```python
from build123d import *


with BuildPart() as part:
    # Esquisse1 → Révolution1 (revolve)
    with BuildSketch(Plane.XY):
        with BuildLine():
            Line((143.396454905, 12.7), (142.494, 12.7))
            Line((142.494, 12.7), (142.494, 0))
            Line((142.494, 0), (130.048, 0))
            Line((130.048, 0), (130.048, 38.1))
            Line((130.048, 38.1), (155.956, 38.1))
            Line((155.956, 38.1), (155.956, 17.260162249))
            Line((155.956, 17.260162249), (149.676227452, 17.260162249))
            ThreePointArc((149.676227452, 17.260162249), (145.79580792, 15.999865109), (143.396454905, 12.7))
        make_face()
    revolve(axis=Axis((0, 0, 0), (0, 1, 0)))


solid = part.part
```
CAD build for the part. Positions are in the model's coordinates, mm. Coordinates: 2 decimals unless noted, no trailing zeros. Order: outer loops, then holes, each group sorted by start corner. A loop starts at its lowest first (then second) coordinate and runs counter-clockwise, first axis right, second up. Notation, with made-up numbers: (-30, 24) - (7, 24) arc R22 cw to (7, 45) - close; hole circle Ø3 at (-33.75, 38.5). An arc over 180 degrees is marked (long way). Use a Markdown table: item, result. Add a question column.
(1) Saw through at B-B (x = 0). Give the cut face in (y, z).
(2) Pull direction Z, two halves, no side cores. Call faces 1 (the face through (-139, 17.26, -58)), 2 (the face through (-30.89, 6.261, 139.106)), 3 (the face through (-28, 19, 127)): +Z half, -Z half, draft (parallel to the pull), parting line (faces both ways), or undercut.
(3) Saw through at A-A (z = 0). Give the cut face in (x, y), then the cut area to 3 significant figures.
(4) Flat gauge pins, fed straight in: pin 1 (10 mm diameter, centred on x = -65.5, y = 4, fed in from -Z); pin 2 (10 mm diameter, centred on y = 15, z = 21.5, fed in from +X); pin 3 (5 mm diameter, centred on y = 16, z = 58, fed in from +X). Where does each tip first touch, or does it go through?
(5) Saw through at D-D (y = 23.5). Give the cut face in (x, z), then the cut area to 3 significant figures.
(6) Saw through at C-C (y = 7). Give the cut face in (x, z), then the cut area to 3 significant figures.
(7) Drill centre lines: line 1 along Z through (x, y) = (1, 12); line 2 along X through (y, z) = (23, 0). Where is each one in solid material? Low to high. Write a range as [from, to].
Solved:
| question | item | result |
|---|---|---|
| 1 | outline | (0, -142.49) - (12.7, -142.49) - (12.7, -143.4) arc R6.6 cw to (17.26, -149.68) - (17.26, -155.96) - (38.1, -155.96) - (38.1, -130.05) - (0, -130.05) - close; (0, 130.05) - (38.1, 130.05) - (38.1, 155.96) - (17.26, 155.96) - (17.26, 149.68) arc R6.6 cw to (12.7, 143.4) - (12.7, 142.49) - (0, 142.49) - close |
| 2 | face 1 | draft |
| 2 | face 2 | parting line |
| 2 | face 3 | undercut |
| 3 | outline | (-155.96, 17.26) - (-149.68, 17.26) arc R6.6 cw to (-143.4, 12.7) - (-142.49, 12.7) - (-142.49, 0) - (-130.05, 0) - (-130.05, 38.1) - (-155.96, 38.1) - close; (130.05, 0) - (142.49, 0) - (142.49, 12.7) - (143.4, 12.7) arc R6.6 cw to (149.68, 17.26) - (155.96, 17.26) - (155.96, 38.1) - (130.05, 38.1) - close |
| 3 | area | 1,530 mm² |
| 4 | pin 1 | stops at z = -129.01 |
| 4 | pin 2 | stops at x = 155.02 |
| 4 | pin 3 | stops at x = 145.62 |
| 5 | outline | circle Ø311.91 at (0, 0); hole circle Ø260.1 at (0, 0) |
| 5 | area | 23,300 mm² |
| 6 | outline | circle Ø284.99 at (0, 0); hole circle Ø260.1 at (0, 0) |
| 6 | area | 10,700 mm² |
| 7 | line 1 | z = [-142.49, -130.04], [130.04, 142.49] |
| 7 | line 2 | x = [-155.96, -130.05], [130.05, 155.96] |
